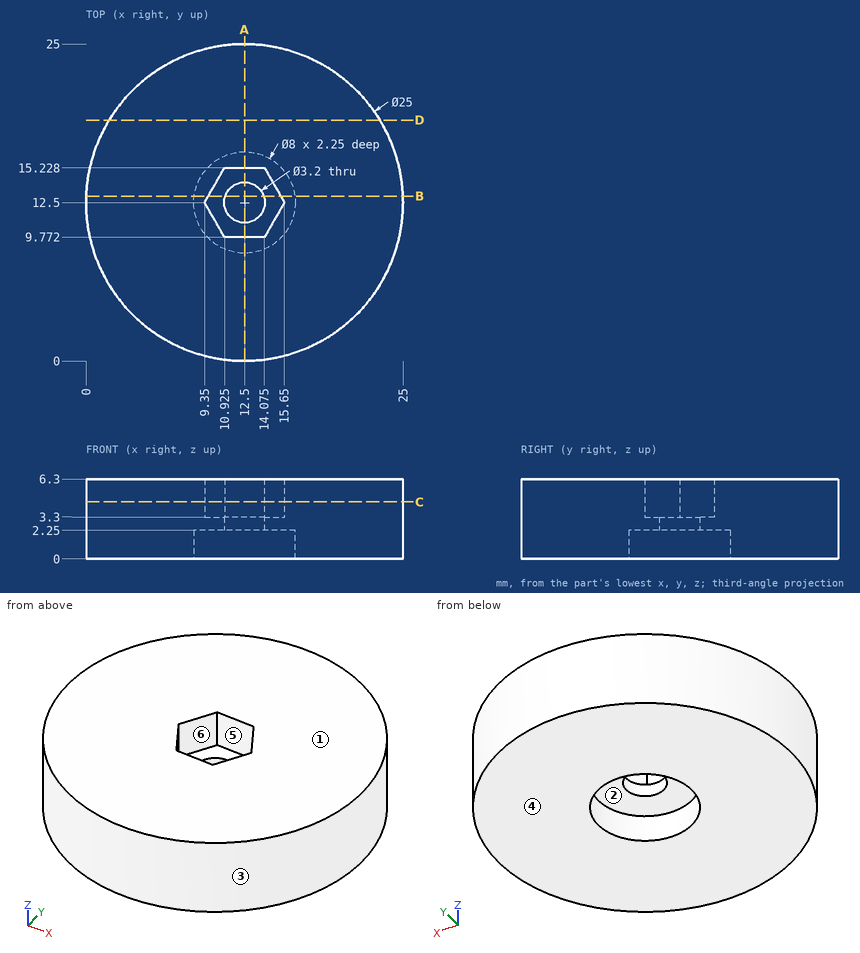
Print and shaded views of the part. All mm, measured from the part's lowest x, y and z. A direction names the side the tool comes from. Coordinates: 2 decimals unless noted, no trailing zeros. Write each loop counter-clockwise with the first axis right and the second up, starting at its lowest first coordinate (ties: lowest second). Pieces come first, ordered by that corner, then holes.
(1) 3-axis set-ups, long thin cutter, end or side, ignore diameter. For the marked faces 1 and 2: which of +Z, -Z, +X, -X, +Y, -Y reach the whole face in a straight line?
(2) Cut at D-D, the plane y = 19. List the corners of the cut face in (x, z), and give its area (3 significant figures).
(3) Cut at B-B, the plane y = 13. List the corners of the cut face in (x, z), and give its area (3 significant figures).
(4) Cut at C-C, the plane z = 4.5. List the corners of the cut face in (x, y) (3 decimals).
(5) Cut at A-A, the plane x = 12.5. List the corners of the cut face in (y, z), and give its area (3 significant figures).
(6) Drill centre lines: probe 1 along X at (y, z) = (12.5, 0.9); probe 2 along X at (y, z) = (12.5, 2.65). Where is each one in solid material? Low to high.
(7) Flat gauge pins, fed straight in: pin 1 (4 mm diameter, centred on x = 11, y = 11, fed in from -Z); pin 2 (2.5 mm diameter, centred on x = 12.5, y = 12.5, fed in from +Z); pin 3 (4.5 mm diameter, centred on x = 13, y = 12.5, fed in from +Z); pin 4 (1 mm diameter, centred on y = 21, z = 1.5, fed in from +X). Where does each tip first touch, or does it go through?
(8) Two-plate mould, pull along X, no slides. Class the marked faces 3, 4, 5 and 6: +X half, -X half, draft (parallel to the pull), parting line (faces both ways), or undercut.
Geometry says:
1. face 1: +Z, +X, -X, +Y, -Y
1. face 2: -Z
2. outline: (1.82, 0) - (23.18, 0) - (23.18, 6.3) - (1.82, 6.3) - close
2. area: 135 mm2
3. outline: (0.01, 0) - (8.53, 0) - (8.53, 2.25) - (10.98, 2.25) - (10.98, 3.3) - (9.64, 3.3) - (9.64, 6.3) - (0.01, 6.3) - close; (14.02, 2.25) - (16.47, 2.25) - (16.47, 0) - (24.99, 0) - (24.99, 6.3) - (15.36, 6.3) - (15.36, 3.3) - (14.02, 3.3) - close
3. area: 119 mm2
4. outline: circle Ø25 at (12.5, 12.5); hole (9.35, 12.5) - (10.925, 9.772) - (14.075, 9.772) - (15.65, 12.5) - (14.075, 15.228) - (10.925, 15.228) - close
5. outline: (0, 0) - (8.5, 0) - (8.5, 2.25) - (10.9, 2.25) - (10.9, 3.3) - (9.77, 3.3) - (9.77, 6.3) - (0, 6.3) - close; (14.1, 2.25) - (16.5, 2.25) - (16.5, 0) - (25, 0) - (25, 6.3) - (15.23, 6.3) - (15.23, 3.3) - (14.1, 3.3) - close
5. area: 120 mm2
6. probe 1: x = 0 to 8.5, 16.5 to 25
6. probe 2: x = 0 to 10.9, 14.1 to 25
7. pin 1: stops at z = 0
7. pin 2: passes through
7. pin 3: stops at z = 3.3
7. pin 4: stops at x = 22.1
8. face 3: parting line
8. face 4: draft
8. face 5: undercut
8. face 6: undercut
